CAD build for the part. Positions are in the model's coordinates, mm. A direction names the side the tool comes from. Round coordinates to 2 decimals unless told otherwise and drop trailing zeros. Write each loop counter-clockwise with the first axis right and the second up, starting at its lowest first coordinate (ties: lowest second). Pieces come first, ordered by that corner, then holes. Notation, with made-up numbers: (26.25, 24.25) - (51.25, 24.25) arc R26 ccw to (51.25, 51.25) - close; hole circle Ø3 at (18, -1). An arc over 180 degrees is marked (long way). Put each result on its own line as item: value. Start each with the question number.
Item 1: Drill centre lines: line 1 (Z direction, x = 63, y = -2.5) (3 decimals); line 2 (X direction, y = -0.6, z = 54); line 3 (Z direction, x = 0, y = -1.45) (3 decimals). Where is each one in solid material? Low to high. Write a range as from..to.
Item 2: 3-axis set-ups, long thin cutter, end or side, ignore diameter. For faces 1 (the cylindrical face through (-54.308, -1.821, -54.156)), 2 (the flat face through (-1, -2, 71.125)): which of +Z, -Z, +X, -X, +Y, -Y reach the whole face in a straight line?
Item 3: Cut at A-A (z = -5.75). Give the cut face in (x, y).
Item 4: Cut at C-C (y = -1.4). Give the cut face in (x, z) (3 decimals).
Item 5: Cut at B-B (x = 0). Give the cut face in (y, z) (3 decimals), and give its area (3 significant figures).
Item 6: Pin check, flat tip, straight feed: pin 1 Ø2.5 at (x, z) = (-55, -52.825) entering from -Y. Stop position of the tip, or through.
```python
from build123d import *

# Parameters (mm, degrees)
F0_W     = 140
F0_H     = 142.25
F0_R     = 56
F1_DEPTH = 3.3
F2_R     = 1.5
F3_DEPTH = 3


with BuildPart() as f1:
    # F0 (on Front) → F1 (new body)
    with BuildSketch(Plane.XZ):
        Rectangle(F0_W, F0_H)
        with Locations((0, -5.75)):
            Circle(F0_R, mode=Mode.SUBTRACT)
    extrude(amount=F1_DEPTH)

    # F2 (on face) → F3 (cut)
    with BuildSketch(Plane.XZ.offset(3.3)):
        with Locations((63, 52.825)):
            Circle(F2_R)
        with Locations((-55, 52.825)):
            Circle(F2_R)
        with Locations((-55, -52.825)):
            Circle(F2_R)
        with Locations((63, -52.825)):
            Circle(F2_R)
    extrude(amount=-F3_DEPTH, mode=Mode.SUBTRACT)


solid = f1.part
```
Output values:
1. line 1: -71.125..-54.325, -51.325..51.325, 54.325..71.125
1. line 2: -70..-55.93, -54.07..62.07, 63.93..70
1. line 3: -71.125..-61.75, 50.25..71.125
2. face 1: -Y
2. face 2: +Z, +X, -X, +Y, -Y
3. outline: (-70, -3.3) - (-56, -3.3) - (-56, 0) - (-70, 0) - close; (56, -3.3) - (70, -3.3) - (70, 0) - (56, 0) - close
4. outline: (-70, -71.125) - (70, -71.125) - (70, 71.125) - (-70, 71.125) - close; hole circle Ø3 at (-55, -52.825); hole circle Ø3 at (-55, 52.825); hole circle Ø112 at (0, -5.75); hole circle Ø3 at (63, -52.825); hole circle Ø3 at (63, 52.825)
5. outline: (-3.3, -71.125) - (0, -71.125) - (0, -61.75) - (-3.3, -61.75) - close; (-3.3, 50.25) - (0, 50.25) - (0, 71.125) - (-3.3, 71.125) - close
5. area: 99.8 mm2
6. pin 1: y = -0.3
